```python
from build123d import *

# Parameters (mm, degrees)
SKETCH1_W           = 177.8
SKETCH1_H           = 114.3
BOSS_EXTRUDE1_DEPTH = 0.254
SKETCH2_R           = 1.143
SKETCH2_W           = 12.7
SKETCH2_H           = 3.175
CUT_EXTRUDE1_DEPTH  = 1.254
SKETCH3_R           = 1.375
SKETCH3_R_2         = 1.5875
SKETCH3_W           = 3.556
SKETCH3_H           = 6.604
CUT_EXTRUDE2_DEPTH  = 1.254


with BuildPart() as part:
    # Sketch1 → Boss-Extrude1 (new body)
    with BuildSketch(Plane(origin=(0, 0, 0), x_dir=(1, 0, 0), z_dir=(0, 1, 0))):
        Rectangle(SKETCH1_W, SKETCH1_H)
    extrude(amount=BOSS_EXTRUDE1_DEPTH)

    # Sketch2 → Cut-Extrude1 (cut, through all)
    with BuildSketch(Plane(origin=(0, 0.254, 0), x_dir=(1, 0, 0), z_dir=(0, 1, 0))):
        with Locations((-57.912, -33.655)):
            Circle(SKETCH2_R)
        with Locations((-50.292, -33.655)):
            Circle(SKETCH2_R)
        with Locations((-50.292, 33.655)):
            Circle(SKETCH2_R)
        with Locations((-57.912, 33.655)):
            Circle(SKETCH2_R)
        with Locations((69.85, -55.5625)):
            Rectangle(SKETCH2_W, SKETCH2_H)
        with Locations((44.45, -55.5625)):
            Rectangle(SKETCH2_W, SKETCH2_H)
        with Locations((19.05, -55.5625)):
            Rectangle(SKETCH2_W, SKETCH2_H)
        with Locations((-6.35, -55.5625)):
            Rectangle(SKETCH2_W, SKETCH2_H)
        with Locations((-31.75, -55.5625)):
            Rectangle(SKETCH2_W, SKETCH2_H)
        with Locations((-57.15, -55.5625)):
            Rectangle(SKETCH2_W, SKETCH2_H)
        with Locations((69.85, 55.5625)):
            Rectangle(SKETCH2_W, SKETCH2_H)
        with Locations((44.45, 55.5625)):
            Rectangle(SKETCH2_W, SKETCH2_H)
        with Locations((19.05, 55.5625)):
            Rectangle(SKETCH2_W, SKETCH2_H)
        with Locations((-6.35, 55.5625)):
            Rectangle(SKETCH2_W, SKETCH2_H)
        with Locations((-31.75, 55.5625)):
            Rectangle(SKETCH2_W, SKETCH2_H)
        with Locations((-57.15, 55.5625)):
            Rectangle(SKETCH2_W, SKETCH2_H)
    extrude(amount=-CUT_EXTRUDE1_DEPTH, mode=Mode.SUBTRACT)

    # Sketch3 → Cut-Extrude2 (cut, through all)
    with BuildSketch(Plane(origin=(0, 0.254, 0), x_dir=(1, 0, 0), z_dir=(0, 1, 0))):
        with Locations((70.976500958, -38.327807122)):
            Circle(SKETCH3_R)
        with Locations((21.976500958, -38.327807122)):
            Circle(SKETCH3_R)
        with Locations((21.976500958, 19.672192878)):
            Circle(SKETCH3_R)
        with Locations((70.976500958, 19.672192878)):
            Circle(SKETCH3_R)
        with Locations((-70.786531145, -24.13)):
            Circle(SKETCH3_R_2)
        with Locations((-70.786531145, 24.13)):
            Circle(SKETCH3_R_2)
        with Locations((-19.989071209, -23.622)):
            Circle(SKETCH3_R_2)
        with Locations((-19.989071209, 1.778)):
            Circle(SKETCH3_R_2)
        with Locations((-82.380316409, 18.923)):
            Rectangle(SKETCH3_W, SKETCH3_H)
        with Locations((-82.380316409, -18.923)):
            Rectangle(SKETCH3_W, SKETCH3_H)
    extrude(amount=-CUT_EXTRUDE2_DEPTH, mode=Mode.SUBTRACT)


solid = part.part
```
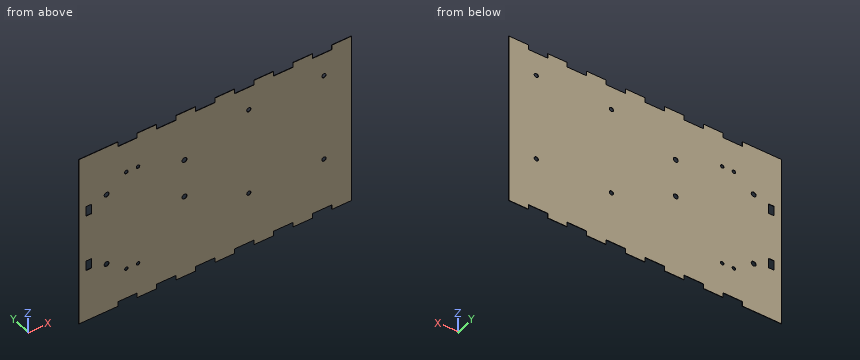
Check sheet for the modelled part. Datum: model origin and axes. Units: mm. Give positions to 0.01 mm unless a question says otherwise; leave off trailing zeros. Write each loop counter-clockwise with the first axis right and the second up, starting at its lowest first coordinate (ties: lowest second). Pieces come first, ordered by that corner, then holes. Notation, with made-up numbers: (42.25, 6.25) - (83.25, 6.25) arc R15 ccw to (83.25, 22.25) - close; hole circle Ø1 at (22, 82). An arc over 180 degrees is marked (long way). Answer as a JSON object with one key per item and string values. Group by question number.
1) Sectioned sample at A-A (x = -36). Record the cut outline in (y, z) (3 decimals), then the cut area to 3 significant figures.
2) Sectioned sample at B-B (y = 0.15). Give the number of separate pieces and of enclosed holes in the cut face, then the cut area to 3 significant figures.
3) Thickness scan on probe 1 along Z at (x, y) = (-58, 0.2) (3 decimals); probe 2 along X at (y, z) = (0.05, -22); probe 3 along Z at (x, y) = (-9, 0.05) (3 decimals). Record the ranges inside material, lowest first. Write a range as from..to.
Geometry results:
{
 "1": {"outline": "(0, -53.975) - (0.254, -53.975) - (0.254, 53.975) - (0, 53.975) - close", "area": "27.4 mm^2"},
 "2": {"separate pieces": "1", "enclosed holes": "14", "area": "19,700 mm^2"},
 "3": {"probe 1": "z = -53.975..-34.795, -32.515..32.515, 34.795..53.975", "probe 2": "x = -88.9..-84.16, -80.6..88.9", "probe 3": "z = -53.975..53.975"}
}
